Design review of the part built by this model. Coordinates are the model's own, in mm. Face numbers are marked on the shaded views. A direction names the side the tool comes from. Coordinates: 2 decimals unless noted, no trailing zeros. Order: outer loops, then holes, each group sorted by start corner. A loop starts at its lowest first (then second) coordinate and runs counter-clockwise, first axis right, second up.
from build123d import *

# Parameters (mm, degrees)
F0_R     = 50.8
F1_DEPTH = 127
F2_DEPTH = 101.6
F4_DEPTH = 25.4


# Not quite as in the source:
# - a feature of the source that left no trace in its solid (it failed there, or was rolled back) is left out


with BuildPart() as f1:
    # F0 (on Front) → F1 (new body)
    with BuildSketch(Plane.XZ):
        with BuildLine():
            ThreePointArc((-61.2979337454, -96.1375838272), (-1.3713712696, -77.6852401135), (24.4270662546, -20.5352401135))
            ThreePointArc((24.4270662546, -20.5352401135), (24.2670376819, -15.5993769332), (23.7876241198, -10.6842454887))
            ThreePointArc((23.7876241198, -10.6842454887), (-51.7729337454, 55.6647598865), (-127.3334916106, -10.6842454887))
            ThreePointArc((-127.3334916106, -10.6842454887), (-119.2731253406, -55.8929003106), (-86.6979337454, -88.260304713))
            ThreePointArc((-86.6979337454, -88.260304713), (-74.3442320368, -93.3155705156), (-61.2979337454, -96.1375838272))
        make_face()
        with Locations((-51.7729337454, -20.5352401135)):
            Circle(F0_R, mode=Mode.SUBTRACT)
    extrude(amount=F1_DEPTH)

    # F0 (on Front) → F2 (join)
    with BuildSketch(Plane.XZ):
        with BuildLine():
            ThreePointArc((-86.6979337454, -88.260304713), (-119.2731253406, -55.8929003106), (-127.3334916106, -10.6842454887))
            Line((-127.3334916106, -10.6842454887), (-200.9979337454, -223.7352401135))
            Line((-200.9979337454, -223.7352401135), (-86.6979337454, -223.7352401135))
            Line((-86.6979337454, -223.7352401135), (-86.6979337454, -88.260304713))
        make_face()
    extrude(amount=F2_DEPTH)

    # F0 (on Front) → F4 (join)
    with BuildSketch(Plane.XZ):
        with BuildLine():
            Line((-61.2979337454, -223.7352401135), (-61.2979337454, -96.1375838272))
            ThreePointArc((-61.2979337454, -96.1375838272), (-74.3442320368, -93.3155705156), (-86.6979337454, -88.260304713))
            Line((-86.6979337454, -88.260304713), (-86.6979337454, -223.7352401135))
            Line((-86.6979337454, -223.7352401135), (-61.2979337454, -223.7352401135))
        make_face()
    extrude(amount=F4_DEPTH)


solid = f1.part
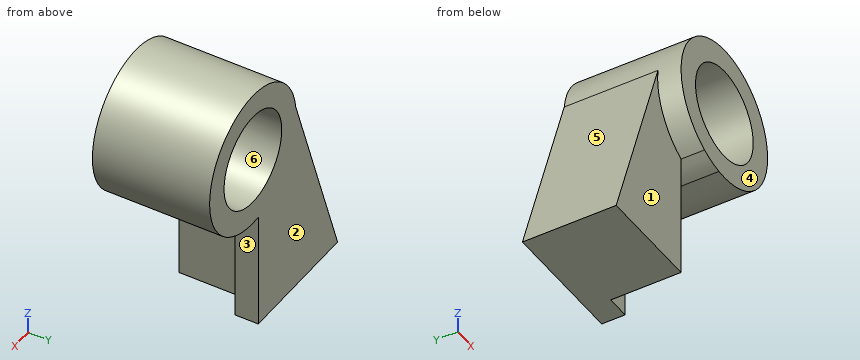
1. Add section A-A (z = -47). Give the boundary of the cut face in (x, y).
2. Insertion check: pin 1 (6 mm diameter, centred on x = -11, y = -86, fed in from +Z); pin 2 (2 mm diameter, centred on y = -87.5, z = -30, fed in from -X); pin 3 (5 mm diameter, centred on y = -70, z = -103.5, fed in from -X); pin 4 (10 mm diameter, centred on x = -52, z = -109, fed in from -Y). Each pin has a flat end and moves straight along its axis. Give the tip position at first contact, or say it passes through.
3. Add section C-C (y = -12). Give the boundary of the cut face in (x, z).
4. To check wall thickness, follow line 1 (Y direction, x = -91.5, z = -203); line 2 (Z direction, x = -40, y = -85); line 3 (Z direction, x = -84, y = -58.5). State the ranges of each line that lie inside material, in increasing order.
5. For the marked faces 1, 2 and 3, list the 3-axis set-ups (+Z, -Z, +X, -X, +Y, -Y) from which the entire face can be reached by the end or side of a thin tool; tool diameter is ignored.
6. Add section D-D (z = -186). Give the boundary of the cut face in (x, y), and give its area (3 significant figures).
7. Mouldability with a two-part tool opening along X and no side actions: class the marked faces 4, 5 and 6 as pulls with the +X half, pulls with the -X half, needs draft (parallel to the pull), parting line crosses it, or undercut.
8. Add section B-B (x = -81.5). Give the boundary of the cut face in (y, z), and give its area (3 significant figures).
Solution:
1. outline: (-139.89, -101.6) - (-123.23, -101.6) - (-123.23, -127) - (-95.13, -127) - (-95.13, 0) - (-139.89, 0) - close; (-8.41, -127) - (19.68, -127) - (19.68, 0) - (-8.41, 0) - close
2. pin 1: stops at z = 45.64
2. pin 2: stops at x = -134.36
2. pin 3: stops at x = -160.29
2. pin 4: passes through
3. outline: (-201, -223.74) - (-61.3, -223.74) - (-61.3, -96.14) arc R76.2 ccw (long way) to (-127.33, -10.68) - close; hole circle Ø101.6 at (-51.77, -20.54)
4. line 1: y = -101.6 to 0
4. line 2: z = -95.82 to -69.95, 28.88 to 54.75
4. line 3: z = -89.58 to -59.8, 18.73 to 48.51
5. face 1: -Z, -X, -Y
5. face 2: +Z, -Z, +X, -X, +Y
5. face 3: -Z, +X, +Y, -Y
6. outline: (-187.95, -101.6) - (-86.7, -101.6) - (-86.7, -25.4) - (-61.3, -25.4) - (-61.3, 0) - (-187.95, 0) - close
6. area: 10,900 mm2
7. face 4: needs draft
7. face 5: pulls with the -X half
7. face 6: undercut
8. outline: (-127, -90.7) - (-25.4, -90.7) - (-25.4, -223.74) - (0, -223.74) - (0, -61.73) - (-127, -61.73) - close; (-127, 20.66) - (0, 20.66) - (0, 49.63) - (-127, 49.63) - close
8. area: 10,700 mm2
